Input: part model. Units: mm. Frame: model coordinates. Round coordinates to 2 decimals unless told otherwise and drop trailing zeros. Order: outer loops, then holes, each group sorted by start corner. A loop starts at its lowest first (then second) coordinate and runs counter-clockwise, first axis right, second up. Notation, with made-up numbers: (62.25, 20) -> (112.25, 20) arc R6 cw to (112.25, 25) -> close; hole circle Ø6 at (-22.75, 39). An arc over 180 degrees is marked (long way). Answer as CSV lines item,"result". Start each with the question number.
1) First-contact query: P1, Ø10, axis at y = -1, z = 6.5, coming from the -X side; P2, Ø10, axis at y = -7.5, z = 14.5, coming from the -X side; P3, Ø1.2, axis at y = -7, z = 19, coming from the -X side; P4, Ø9.5, axis at y = -1, z = 20.5, coming from the +X side. Flat tips, straight axial feed; report the tip coordinate or a pass-through.
2) Section query A-A, the plane y = -1.25. Output: boundary loops of the cut face in (x, z).
3) Line query: L1, parallel to Y at x = 0.15, z = 4; L2, parallel to X at y = -8.25, z = 8; L3, parallel to Z at x = -3.35, y = -7. Output: solid intervals per line, ascending.
4) Section query B-B, the plane z = 19. Output: boundary loops of the cut face in (x, y), and give its area (3 significant figures).
5) Section query C-C, the plane z = 8.5. Output: boundary loops of the cut face in (x, y), and give its area (3 significant figures).
6) Mould query, pull axis Y, two halves, no side actions, for faces 1 (the face through (-3.494, -7.217, 18.024)), 2 (the face through (-3.506, -9.715, 23.699)), 3 (the face through (-3, 0, 20)). Classes: +Y half, -Y half, draft (parallel to the pull), parting line (faces both ways), or undercut.
```python
from build123d import *

# Parameters (mm, degrees)
F1_DEPTH = 10
F2_R     = 5
F3_R     = 1
F4_DEPTH = 25
F5_R     = 1
F7_DEPTH = 1
F8_R     = 0.2
F9_SIZE  = 0.1


with BuildPart() as f1:
    # F0 (on Front) → F1 (new body, symmetric)
    with BuildSketch(Plane.XZ):
        with BuildLine():
            Line((0, 9.1715728753), (0, 0))
            Line((0, 0), (1, 0))
            Line((1, 0), (1, 9.1715728753))
            ThreePointArc((1, 9.1715728753), (0.7716385975, 10.3196231723), (0.1213203436, 11.2928932188))
            Line((0.1213203436, 11.2928932188), (-2.4142135624, 13.8284271247))
            ThreePointArc((-2.4142135624, 13.8284271247), (-2.847759065, 14.4772738224), (-3, 15.2426406871))
            Line((-3, 15.2426406871), (-3, 24))
            Line((-3, 24), (-4, 24))
            Line((-4, 24), (-4, 15.2426406871))
            ThreePointArc((-4, 15.2426406871), (-3.7716385975, 14.09459039), (-3.1213203436, 13.1213203436))
            Line((-3.1213203436, 13.1213203436), (-0.5857864376, 10.5857864376))
            ThreePointArc((-0.5857864376, 10.5857864376), (-0.152240935, 9.93693974), (0, 9.1715728753))
        make_face()
    extrude(amount=F1_DEPTH, both=True)

    # F2
    f2_edges = [f1.edges().sort_by_distance(p)[0] for p in [
        (0.5, -10, 0),
        (0.5, 10, 0),
    ]]
    fillet(f2_edges, radius=F2_R)

    # F3 (on face) → F4 (cut)
    with BuildSketch(Plane.YZ.offset(-3)):
        with Locations((-7, 19)):
            Circle(F3_R)
        with Locations((7, 19)):
            Circle(F3_R)
    extrude(amount=-F4_DEPTH, mode=Mode.SUBTRACT)

    # F5
    f5_edges = [f1.edges().sort_by_distance(p)[0] for p in [
        (-3.5, -10, 24),
        (-3.5, 10, 24),
    ]]
    fillet(f5_edges, radius=F5_R)

    # F6 (on face) → F7 (cut, through all)
    with BuildSketch(Plane.YZ.offset(1)):
        with BuildLine():
            Line((-4, 2.0857864376), (4, 2.0857864376))
            ThreePointArc((4, 2.0857864376), (4.7071067812, 2.3786796564), (5, 3.0857864376))
            Line((5, 3.0857864376), (5, 7.0857864376))
            Line((5, 7.0857864376), (-5, 7.0857864376))
            Line((-5, 7.0857864376), (-5, 3.0857864376))
            ThreePointArc((-5, 3.0857864376), (-4.7071067812, 2.3786796564), (-4, 2.0857864376))
        make_face()
    extrude(amount=-F7_DEPTH, mode=Mode.SUBTRACT)

    # F8
    f8_edges = [f1.edges().sort_by_distance(p)[0] for p in [
        (0.5, 5, 7.085786),
        (0.5, -5, 7.085786),
    ]]
    fillet(f8_edges, radius=F8_R)

    # F9
    f9_edges = [f1.edges().sort_by_distance(p)[0] for p in [
        (1, 8.535534, 1.464466),
        (1, 0, 7.085786),
        (-3, 6, 19),
        (-3, -8, 19),
        (-4, -8, 19),
        (-4, 6, 19),
        (-3.771639, -10, 14.09459),
        (0, -5, 4.985786),
    ]]
    chamfer(f9_edges, length=F9_SIZE)


solid = f1.part
```
Findings:
1,P1,"stops at x = -1.5"
1,P2,"stops at x = -4"
1,P3,"passes through"
1,P4,"stops at x = -3"
2,outline,"(-4, 15.24) arc R3 ccw to (-3.12, 13.12) -> (-0.59, 10.59) arc R2 cw to (0, 9.17) -> (0, 7.19) -> (0.1, 7.09) -> (0.9, 7.09) -> (1, 7.19) -> (1, 9.17) arc R3 ccw to (0.12, 11.29) -> (-2.41, 13.83) arc R2 cw to (-3, 15.24) -> (-3, 23.9) -> (-3.1, 24) -> (-3.9, 24) -> (-4, 23.9) -> close; (0, 0.1) -> (0.1, 0) -> (0.9, 0) -> (1, 0.1) -> (1, 1.99) -> (0.9, 2.09) -> (0.1, 2.09) -> (0, 1.99) -> close"
3,L1,"y = -9.9 to -5, 5 to 9.9"
3,L2,"x = 0 to 1"
3,L3,"z = 13.38 to 18, 20 to 24"
4,outline,"(-4, -9.9) -> (-3.9, -10) -> (-3.1, -10) -> (-3, -9.9) -> (-3, -8.1) -> (-3.1, -8) -> (-3.9, -8) -> (-4, -8.1) -> close; (-4, -5.9) -> (-3.9, -6) -> (-3.1, -6) -> (-3, -5.9) -> (-3, 5.9) -> (-3.1, 6) -> (-3.9, 6) -> (-4, 5.9) -> close; (-4, 8.1) -> (-3.9, 8) -> (-3.1, 8) -> (-3, 8.1) -> (-3, 9.9) -> (-3.1, 10) -> (-3.9, 10) -> (-4, 9.9) -> close"
4,area,"15.9 mm^2"
5,outline,"(0, -9.9) -> (0.1, -10) -> (0.9, -10) -> (1, -9.9) -> (1, 9.9) -> (0.9, 10) -> (0.1, 10) -> (0, 9.9) -> close"
5,area,"20.0 mm^2"
6,face 1,"undercut"
6,face 2,"-Y half"
6,face 3,"draft"
